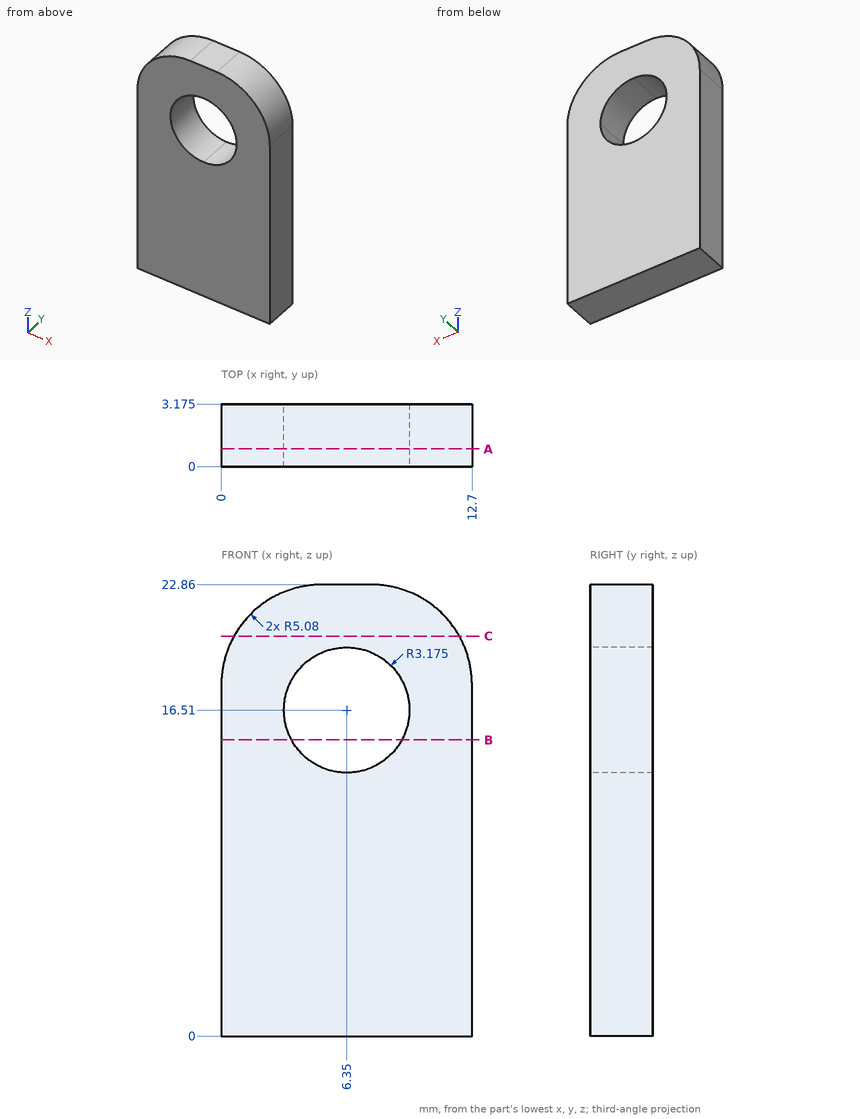
The figure shows three views and two pictorial views of one solid part (mm, origin at its lowest corner). Answer the questions. Coordinates: 2 decimals unless noted, no trailing zeros. Order: outer loops, then holes, each group sorted by start corner. A loop starts at its lowest first (then second) coordinate and runs counter-clockwise, first axis right, second up. Notation, with made-up numbers: (55.25, 78) - (69.25, 78) arc R20 cw to (69.25, 98) - close; hole circle Ø5 at (27.25, 33). An arc over 180 degrees is marked (long way). Answer as a JSON object with one key per item and string values.
1. Find section C-C on z = 20.25. Determine the outline of the cut face in (x, y) (3 decimals).
Output values:
{"outline": "(0.641, 0) - (12.059, 0) - (12.059, 3.175) - (0.641, 3.175) - close"}
2. Each of these flat-tipped pins is pushed along its axis until it touches: P1, Ø1, axis at x = 1.5, y = 0.5, coming from the +Z side; P2, Ø1.5, axis at x = 9.5, y = 1, coming from the +Z side. Where does it stop, or does it pass through?
Output values:
{"P1": "stops at z = 21.82", "P2": "stops at z = 22.73"}
3. Find section A-A on y = 0.9. Determine the outline of the cut face in (x, z) (3 decimals).
Output values:
{"outline": "(0, 0) - (12.7, 0) - (12.7, 17.78) arc R5.08 ccw to (7.62, 22.86) - (5.08, 22.86) arc R5.08 ccw to (0, 17.78) - close; hole circle Ø6.35 at (6.35, 16.51)"}
4. Find section B-B on z = 15. Determine the outline of the cut face in (x, y) (3 decimals), plus the area to 3 significant figures.
Output values:
{"outline": "(0, 0) - (3.557, 0) - (3.557, 3.175) - (0, 3.175) - close; (9.143, 0) - (12.7, 0) - (12.7, 3.175) - (9.143, 3.175) - close", "area": "22.6 mm²"}
5. Consider line 1 (Z direction, x = 6.25, y = 2.4); line 2 (X direction, y = 2.85, z = 14.5); line 3 (Z direction, x = 9, y = 1.8). Determine where each line is inside the solid, lowest interval first.
Output values:
{"line 1": "z = 0 to 13.34, 19.68 to 22.86", "line 2": "x = 0 to 3.89, 8.81 to 12.7", "line 3": "z = 0 to 14.76, 18.26 to 22.67"}
